Geometry: final body of the model. Coordinates: model frame, mm. A direction names the side the tool comes from. Coordinates: 2 decimals unless noted, no trailing zeros. Loops run counter-clockwise (first coordinate to the right, second up) from the corner with the lowest first, then second, coordinate; pieces in that order, holes last. Notation, with made-up numbers: (62, -20.5) - (93, -20.5) arc R16 ccw to (93, -1.5) - close; hole circle Ø2 at (28, 81.5). An arc over 180 degrees is marked (long way). Return JSON: item names as keys, results as strings.
from build123d import *

# Parameters (mm, degrees)
PAD_DEPTH       = 38
POCKET_DEPTH    = 20
FILLET_R        = 4
FILLET001_R     = 4
FILLET002_R     = 3
SKETCH002_W     = 986
SKETCH002_H     = 486
POCKET001_DEPTH = 38.001
FILLET003_R     = 3


with BuildPart() as part:
    # Sketch → Pad (new body)
    with BuildSketch(Plane.XY):
        with BuildLine():
            Line((0, 0), (0, 635))
            Line((0, 635), (1890, 635))
            Line((1890, 635), (1890, 60))
            Line((1890, 60), (1335.710678, 60))
            ThreePointArc((1335.710678, 60), (1316.576507, 56.193977), (1300.355339, 45.355339))
            Line((1255, 0), (1300.355339, 45.355339))
            Line((0, 0), (1255, 0))
        make_face()
    extrude(amount=PAD_DEPTH)

    # Sketch001 (on Face8 of Pad) → Pocket (cut)
    with BuildSketch(Plane(origin=(0, 0, 0), x_dir=(1, 0, 0), z_dir=(0, 0, -1))):
        Polygon((1535, -60), (1535, -130), (1510, -154.999975), (1510, -190), (1570, -190), (1570, -154.999975), (1545, -130), (1545, -60), align=None)
        Polygon((1710, -60), (1710, -130), (1685, -154.999975), (1685, -190), (1745, -190), (1745, -154.999975), (1720, -130), (1720, -60), align=None)
        Polygon((1360, -60), (1360, -130), (1335, -155), (1335, -190), (1395, -190), (1395, -155), (1370, -130), (1370, -60), align=None)
    extrude(amount=-POCKET_DEPTH, mode=Mode.SUBTRACT)

    # Fillet
    fillet_edges = [part.edges().sort_by_distance(p)[0] for p in [
        (1510, 154.999975, 10),
        (1510, 190, 10),
        (1570, 190, 10),
        (1570, 154.999975, 10),
    ]]
    fillet(fillet_edges, radius=FILLET_R)

    # Fillet001
    fillet001_edges = [part.edges().sort_by_distance(p)[0] for p in [
        (1685, 154.999975, 10),
        (1685, 190, 10),
        (1745, 154.999975, 10),
        (1745, 190, 10),
    ]]
    fillet(fillet001_edges, radius=FILLET001_R)

    # Fillet002
    fillet002_edges = [part.edges().sort_by_distance(p)[0] for p in [
        (1335, 155, 10),
        (1335, 190, 10),
        (1395, 155, 10),
        (1395, 190, 10),
    ]]
    fillet(fillet002_edges, radius=FILLET002_R)

    # Sketch002 (on Face41 of Fillet001) → Pocket001 (cut, through all)
    with BuildSketch(Plane.XY.offset(38)):
        with Locations((620, 317.5)):
            Rectangle(SKETCH002_W, SKETCH002_H)
    extrude(amount=-POCKET001_DEPTH, mode=Mode.SUBTRACT)

    # Fillet003
    fillet003_edges = [part.edges().sort_by_distance(p)[0] for p in [
        (1113, 74.5, 19),
        (127, 560.5, 19),
        (127, 74.5, 19),
        (1113, 560.5, 19),
    ]]
    fillet(fillet003_edges, radius=FILLET003_R)


solid = part.part
Item 1: Reachability of faces 1 (the face through (1365, 153, 20)), 2 (the face through (1168, 322, 38)), 3 (the face through (1113, 314, 19)) from +Z, -Z, +X, -X, +Y, -Y: full face, straight path, thin tool, end or side. Return the list, or none.
Worked out:
{"face 1": "-Z", "face 2": "+Z, +X, -X, +Y, -Y", "face 3": "+Z, -Z"}
Item 2: Section query B-B, the plane x = 184. Return loops of the section in (y, z), and give its area (3 significant figures).
Worked out:
{"outline": "(0, 0) - (74.5, 0) - (74.5, 38) - (0, 38) - close; (560.5, 0) - (635, 0) - (635, 38) - (560.5, 38) - close", "area": "5,660 mm^2"}
Item 3: Ray query, probe 1 along X at (y, z) = (459, 19); probe 2 along Y at (x, z) = (504, 32.5); probe 3 along Y at (x, z) = (1778.5, 8). Return the intervals inside material, ascending. Write a range as from..to.
Worked out:
{"probe 1": "0..127, 1113..1890", "probe 2": "0..74.5, 560.5..635", "probe 3": "60..635"}
Item 4: Section query A-A, the plane y = 276. Return loops of the section in (x, z).
Worked out:
{"outline": "(0, 0) - (127, 0) - (127, 38) - (0, 38) - close; (1113, 0) - (1890, 0) - (1890, 38) - (1113, 38) - close"}
Item 5: First-contact query: pin 1 Ø22 at (x, z) = (1710, 13) entering from -Y. Flat tip, straight axial feed; report the tip coordinate or a pass-through.
Worked out:
{"pin 1": "y = 60"}
Item 6: Mould query, pull axis Y, two halves, no side actions, for faces 4 (the face through (1890, 352, 19)), 5 (the face through (932, 635, 19)), 6 (the face through (613, 560.5, 19)), 7 (the face through (1617, 60, 19)). Classes: +Y half, -Y half, draft (parallel to the pull), parting line (faces both ways), or undercut.
Worked out:
{"face 4": "draft", "face 5": "+Y half", "face 6": "undercut", "face 7": "-Y half"}
Item 7: Section query C-C, the plane z = 31.5. Return loops of the section in (x, y), and give its area (3 significant figures).
Worked out:
{"outline": "(0, 0) - (1255, 0) - (1300.36, 45.36) arc R50 cw to (1335.71, 60) - (1890, 60) - (1890, 635) - (0, 635) - close; hole (127, 77.5) arc R3 ccw to (130, 74.5) - (1110, 74.5) arc R3 ccw to (1113, 77.5) - (1113, 557.5) arc R3 ccw to (1110, 560.5) - (130, 560.5) arc R3 ccw to (127, 557.5) - close", "area": "685,000 mm^2"}
